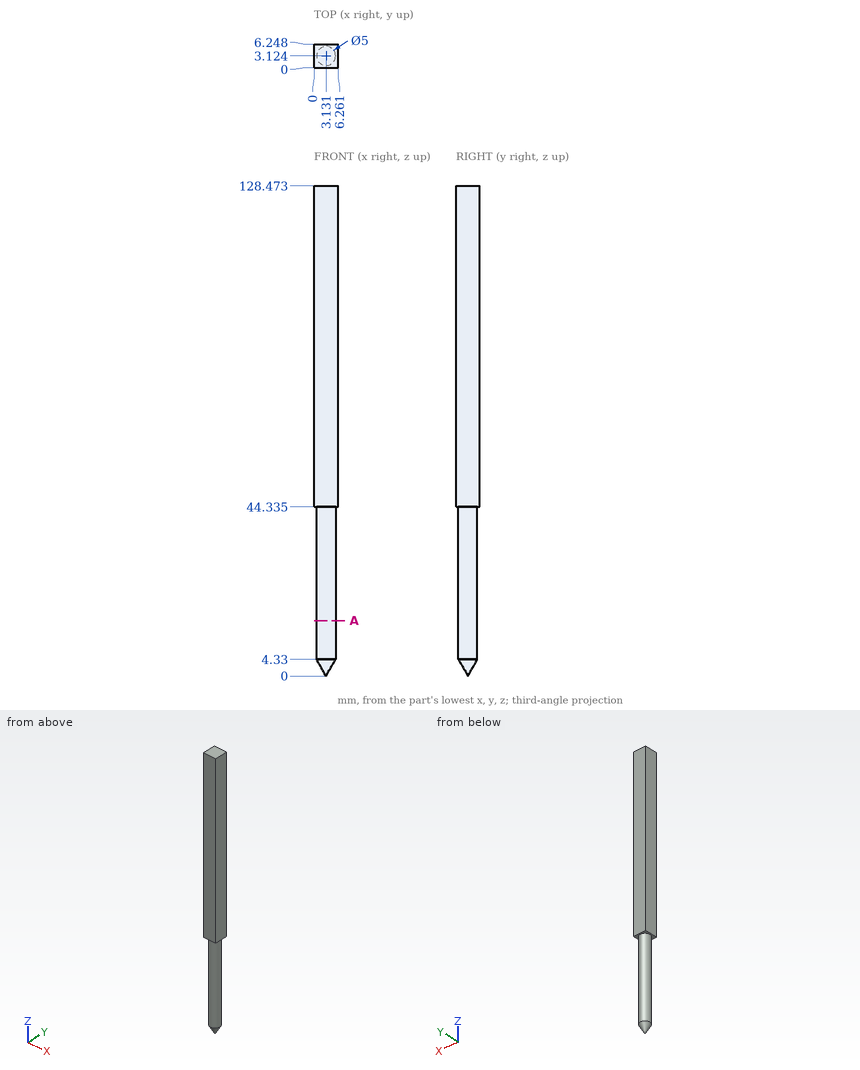
Study the drawing (mm; zero at the part's minimum x, y, z) and answer. Round coordinates to 2 decimals unless told otherwise and drop trailing zeros. Order: outer loops, then holes, each group sorted by start corner. A loop starts at its lowest first (then second) coordinate and runs counter-clockwise, first axis right, second up. Notation, with made-up numbers: (-39.5, -21.5) -> (-5.5, -21.5) arc R26 cw to (-5.5, 13.5) -> close; hole circle Ø3 at (48.25, -3). An arc over 180 degrees is marked (long way). Write each question's results on one line, items separated by ' | '. Start each with the question number.
Q1. Straight lines are drawn through the part: probe 1 along Z at (x, y) = (1, 1.25) (1 decimal); probe 2 along Y at (x, z) = (3.25, 32); probe 3 along Z at (x, y) = (3.25, 1.5) (1 decimal). For each, find the intervals that lie inside material, in ascending order. Write a range as from..to.
Q2. Find section A-A (z = 14.5). Determine the outline of the cut face in (x, y) (1 decimal).
Q3. This flat-tipped pin is pushed along its axis until it touches: pin 1 (3 mm diameter, centred on x = 3, z = 34, fed in from -Y). Where does it stop, or does it pass through?
Worked answers:
1) probe 1: z = 44.3..128.5 | probe 2: y = 0.63..5.62 | probe 3: z = 2.8..128.5
2) outline: circle Ø5 at (3.1, 3.1)
3) pin 1: stops at y = 0.62
